Could you check a few things on this model? Use its own coordinates, in mm. A direction names the side the tool comes from. Give positions to 0.01 mm unless a question says otherwise; leave off trailing zeros. Order: outer loops, then holes, each group sorted by start corner. A loop starts at its lowest first (then second) coordinate and runs counter-clockwise, first axis right, second up. Notation, with made-up numbers: (81, 18) -> (134, 18) arc R26 ccw to (134, 38) -> close; hole circle Ø11 at (68, -17.5). An arc over 180 degrees is marked (long way). One line per item, written item: value.
```python
from build123d import *

# Parameters (mm, degrees)
BOSS_EXTRUDE1_DEPTH = 3.5
BOSS_EXTRUDE2_DEPTH = 1
SKETCH4_R           = 4.75
CUT_EXTRUDE1_DEPTH  = 24.115651093
SKETCH5_W           = 17.56
SKETCH5_H           = 4.5
BOSS_EXTRUDE3_DEPTH = 0.15
SKETCH6_W           = 17.56
SKETCH6_H           = 4.5
BOSS_EXTRUDE4_DEPTH = 7.5
SKETCH9_W           = 8
SKETCH9_H           = 2
CUT_EXTRUDE2_DEPTH  = 1
FILLET1_R           = 1
CUT_EXTRUDE3_REACH  = 30.715
SKETCH10_W          = 6.92
SKETCH10_H          = 1
SKETCH11_W          = 4.5
SKETCH11_H          = 3.588872583
CUT_EXTRUDE4_DEPTH  = 0.25


with BuildPart() as part:
    # Sketch1 → Boss-Extrude1 (new body)
    with BuildSketch(Plane.XY):
        with BuildLine():
            ThreePointArc((14.980604809, 6.55), (8.78, 2), (2.579395191, 6.55))
            Line((2.579395191, 6.55), (0, 6.55))
            Line((0, 6.55), (0, 0))
            Line((0, 0), (17.56, 0))
            Line((17.56, 0), (17.56, 6.55))
            Line((17.56, 6.55), (14.980604809, 6.55))
        make_face()
        with BuildLine():
            ThreePointArc((2.579395191, 6.55), (2.679421093, 10.743420825), (5.32, 14.002581212))
            Line((5.32, 14.002581212), (5.32, 14.619498126))
            ThreePointArc((5.32, 14.619498126), (1.449679407, 11.382680416), (0, 6.55))
            Line((0, 6.55), (2.579395191, 6.55))
        make_face()
        with BuildLine():
            ThreePointArc((12.24, 14.002581212), (14.880578907, 10.743420825), (14.980604809, 6.55))
            Line((14.980604809, 6.55), (17.56, 6.55))
            ThreePointArc((17.56, 6.55), (16.110320593, 11.382680416), (12.24, 14.619498126))
            Line((12.24, 14.619498126), (12.24, 14.002581212))
        make_face()
    extrude(amount=BOSS_EXTRUDE1_DEPTH)

    # Sketch3 → Boss-Extrude2 (add)
    with BuildSketch(Plane.XY.offset(3.5)):
        with BuildLine():
            Line((12.24, 14.619498126), (12.24, 14.002581212))
            ThreePointArc((12.24, 14.002581212), (8.78, 2), (5.32, 14.002581212))
            Line((5.32, 14.002581212), (5.32, 14.619498126))
            ThreePointArc((5.32, 14.619498126), (1.449679407, 11.382680416), (0, 6.55))
            Line((0, 6.55), (0, 0))
            Line((0, 0), (17.56, 0))
            Line((17.56, 0), (17.56, 6.55))
            ThreePointArc((17.56, 6.55), (16.110320593, 11.382680416), (12.24, 14.619498126))
        make_face()
        with BuildLine():
            Line((5.32, 14.619498126), (12.24, 14.619498126))
            Line((12.24, 14.619498126), (12.24, 14.002581212))
            ThreePointArc((12.24, 14.002581212), (8.78, 2), (5.32, 14.002581212))
            Line((5.32, 14.002581212), (5.32, 14.619498126))
        make_face()
    extrude(amount=BOSS_EXTRUDE2_DEPTH)

    # Sketch4 → Cut-Extrude1 (cut, through all)
    with BuildSketch(Plane(origin=(0, 0, 3.5), x_dir=(-1, 0, 0), z_dir=(0, 0, -1))):
        with Locations((-8.78, 8.5)):
            Circle(SKETCH4_R)
    extrude(amount=-CUT_EXTRUDE1_DEPTH, mode=Mode.SUBTRACT)

    # Sketch5 → Boss-Extrude3 (add)
    with BuildSketch(Plane.XZ):
        with Locations((8.78, 2.25)):
            Rectangle(SKETCH5_W, SKETCH5_H)
    extrude(amount=BOSS_EXTRUDE3_DEPTH)

    # Sketch6 → Boss-Extrude4 (add)
    with BuildSketch(Plane.XZ.offset(0.15)):
        with Locations((8.78, 2.25)):
            Rectangle(SKETCH6_W, SKETCH6_H)
    extrude(amount=BOSS_EXTRUDE4_DEPTH)

    # Sketch9 → Cut-Extrude2 (cut)
    with BuildSketch(Plane.XY.offset(4.5)):
        with Locations((8.78, -5.353166831)):
            Rectangle(SKETCH9_W, SKETCH9_H)
    extrude(amount=-CUT_EXTRUDE2_DEPTH, mode=Mode.SUBTRACT)

    # Fillet1
    fillet1_edges = [part.edges().sort_by_distance(p)[0] for p in [
        (4.78, -5.353166831, 4.5),
        (12.78, -5.353166831, 4.5),
        (8.78, -4.353166831, 4.5),
    ]]
    fillet(fillet1_edges, radius=FILLET1_R - 0.0001)  # a hair under: the kernel refuses the full size

    # Sketch10 → Cut-Extrude3 (cut, up to next)
    with BuildSketch(Plane(origin=(0, 14.619498126, 0), x_dir=(1, 0, 0), z_dir=(0, 1, 0)), mode=Mode.PRIVATE) as cut_extrude3_sk1:
        with Locations((8.78, -4)):
            Rectangle(SKETCH10_W, SKETCH10_H)
    cut_extrude3_tool1 = extrude(cut_extrude3_sk1.sketch, amount=-CUT_EXTRUDE3_REACH, mode=Mode.PRIVATE) & part.part
    add(cut_extrude3_tool1.solids().sort_by_distance((8.78, 14.619498, 4))[0], mode=Mode.SUBTRACT)

    # Sketch11 → Cut-Extrude4 (cut)
    with BuildSketch(Plane(origin=(5.32, 0, 0), x_dir=(0, 0, -1), z_dir=(1, 0, 0))):
        with Locations((-2.25, 12.825061835)):
            Rectangle(SKETCH11_W, SKETCH11_H)
    cut_extrude4 = extrude(amount=-CUT_EXTRUDE4_DEPTH, mode=Mode.SUBTRACT)

    # Mirror1: Cut-Extrude4 across plane
    add(cut_extrude4.mirror(Plane.ZY.offset(-8.78)), mode=Mode.SUBTRACT)


solid = part.part
```
1) We'd pull the mould along Y, two halves only. Please class faces 1 (the flat face through (9, -7.65, 2)), 2 (the cylindrical face through (13.081, -5.166, 4.215)), 3 (the flat face through (9, -1, 0)), 4 (the cylindrical face through (16.22, 11.21, 2.22)): +Y half, -Y half, draft (parallel to the pull), parting line (faces both ways), or undercut.
Answer below:
face 1: -Y half
face 2: undercut
face 3: draft
face 4: +Y half
2) For faces 5 (the cylindrical face through (4.479, -5.166, 4.215)), 6 (the flat face through (8.7, 3.6, 3.5)), 7 (the flat face through (12.49, 14, 3)), which set-ups out of +Z, -Z, +X, -X, +Y, -Y let a thin tool reach every point of the face, with its end or its side?
Answer below:
face 5: +Z
face 6: -Z
face 7: +Z, -Z, +Y
3) Suppose I cut it at A-A, the plane z = 2.2. Write out the boundary of the cut face in (x, y), then the cut area to 3 significant figures.
Answer below:
outline: (0, -7.65) -> (17.56, -7.65) -> (17.56, 6.55) arc R8.78 ccw to (12.49, 14.51) -> (12.49, 13.84) arc R6.5 cw (long way) to (5.07, 13.84) -> (5.07, 14.51) arc R8.78 ccw to (0, 6.55) -> close
area: 234 mm2
4) For P1, Ø0.9, axis at y = 13, z = 2, coming from the -X side; P2, Ø0.8, axis at x = 7.5, z = 4, coming from the +Y side; P3, Ø0.6, axis at x = 9, y = -5.5, coming from the +Z side; P4, Ø9.5, axis at x = 6, y = 6, coming from the -Z side, each with a flat end and sliding along its axis, tell me the tip position at first contact or that it passes through.
Answer below:
P1: stops at x = 2.37
P2: stops at y = 4.06
P3: stops at z = 3.5
P4: stops at z = 0
5) Suppose I cut it at B-B, the plane y = 8.5. Write out the boundary of the cut face in (x, z).
Answer below:
outline: (0.22, 0) -> (2.28, 0) -> (2.28, 3.5) -> (4.03, 3.5) -> (4.03, 4.5) -> (0.22, 4.5) -> close; (13.53, 3.5) -> (15.28, 3.5) -> (15.28, 0) -> (17.34, 0) -> (17.34, 4.5) -> (13.53, 4.5) -> close
6) If I drill on line 1 along X through (y, z) = (8.5, 3.85); line 2 along X through (y, z) = (8, 1.2); line 3 along Z through (x, y) = (9.75, 3.5), over which ranges is the centre line in solid material (lowest first)?
Answer below:
line 1: x = 0.22 to 4.03, 13.53 to 17.34
line 2: x = 0.12 to 2.3, 15.26 to 17.44
line 3: z = 3.5 to 4.5
